Input: part model. Units: mm. Frame: model coordinates. A direction names the side the tool comes from. Coordinates: 2 decimals unless noted, no trailing zeros. Write each loop counter-clockwise with the first axis right and the second up, starting at its lowest first coordinate (ties: lowest second). Pieces come first, ordered by that corner, then holes. Notation, with made-up numbers: (30, -26) -> (62, -26) arc R14 ccw to (62, -12) -> close; hole circle Ø6 at (84, 54.5). An arc over 180 degrees is marked (long way). Use one line per item in the form item = value. Start each with the question number.
(1) Set-up query: faces 1 (the face through (-105, 257, 230)), 2 (the face through (95.38, 280.04, 240.14)). Return all of +Z, -Z, +X, -X, +Y, -Y with unobstructed straight access to the full face (end or side cutting, diameter ignored); none if empty.
(2) Cut plane C-C on y = 427. Return the cut outline in (x, z).
(3) Cut plane A-A on x = 0. Return the cut outline in (y, z).
(4) Ray query, line 1 along X through (y, z) = (73, 57); line 2 along Y through (x, z) = (0, 239). Return the intervals inside material, ascending.
(5) Pull-direction query (X, two-part tool) for faces 3 (the face through (-3, 135, -250)), 4 (the face through (230, 257, -3)), 5 (the face through (250, 246, -3)); classes: released by +X, released by -X, zero draft, split by the parting line, or undercut.
(6) Cut plane D-D on z = 116.5. Return the cut outline in (x, y).
(7) Cut plane B-B on y = 250. Return the cut outline in (x, z).
```python
from build123d import *

# Parameters (mm, degrees)
F0_W      = 500
F0_H      = 500
F1_DEPTH  = 500
F2_T      = -20
F3_R      = 100
F4_DEPTH  = 25
F4_FACE_R = 100
F5_DEPTH  = 525.001


with BuildPart() as f1:
    # F0 (on Front) → F1 (new body)
    with BuildSketch(Plane.XZ):
        Rectangle(F0_W, F0_H)
    extrude(amount=-F1_DEPTH)

    # F2
    f2_openings = [f1.faces().sort_by_distance(p)[0] for p in [
        (0, 500, 0),
    ]]
    offset(amount=F2_T, openings=f2_openings)

    # F3 (on face) → F4 (join)
    with BuildSketch(Plane.XY.offset(250)):
        with Locations((0, 250)):
            Circle(F3_R)
    extrude(amount=F4_DEPTH)

    # F4_face (on face) → F5 (cut, through all)
    with BuildSketch(Plane(origin=(0, 250, 275), x_dir=(1, 0, 0), z_dir=(0, 0, 1))):
        Circle(F4_FACE_R)
    extrude(amount=-F5_DEPTH, mode=Mode.SUBTRACT)


solid = f1.part
```
Values:
q1.face_1 = +Y
q1.face_2 = +Z, -Z
q2.outline = (-250, -250) -> (250, -250) -> (250, 250) -> (-250, 250) -> close; hole (-230, -230) -> (230, -230) -> (230, 230) -> (-230, 230) -> close
q3.outline = (0, -250) -> (150, -250) -> (150, -230) -> (20, -230) -> (20, 230) -> (150, 230) -> (150, 250) -> (0, 250) -> close; (350, -250) -> (500, -250) -> (500, -230) -> (350, -230) -> close; (350, 230) -> (500, 230) -> (500, 250) -> (350, 250) -> close
q4.line_1 = -250 to -230, 230 to 250
q4.line_2 = 0 to 150, 350 to 500
q5.face_3 = zero draft
q5.face_4 = undercut
q5.face_5 = released by +X
q6.outline = (-250, 0) -> (250, 0) -> (250, 500) -> (230, 500) -> (230, 20) -> (-230, 20) -> (-230, 500) -> (-250, 500) -> close
q7.outline = (-250, -250) -> (-100, -250) -> (-100, -230) -> (-230, -230) -> (-230, 230) -> (-100, 230) -> (-100, 250) -> (-250, 250) -> close; (100, -250) -> (250, -250) -> (250, 250) -> (100, 250) -> (100, 230) -> (230, 230) -> (230, -230) -> (100, -230) -> close
